Design review of the part built by this model. Coordinates are the model's own, in mm. A direction names the side the tool comes from. Give positions to 0.01 mm unless a question says otherwise; leave off trailing zeros. Order: outer loops, then holes, each group sorted by start corner. A loop starts at its lowest first (then second) coordinate and runs counter-clockwise, first axis right, second up.
```python
from build123d import *

# Parameters (mm, degrees)
SKETCH1_R           = 3.175
BOSS_EXTRUDE1_DEPTH = 20.6
SKETCH2_R           = 19.05
BOSS_EXTRUDE2_DEPTH = 1.6
BOSS_EXTRUDE3_DEPTH = 4.8
BOSS_EXTRUDE4_DEPTH = 51.2
SKETCH7_W           = 3.420526276
SKETCH7_H           = 1.112659396
CUT_EXTRUDE5_DEPTH  = 15
CUT_EXTRUDE6_REACH  = 70.749
SKETCH8_R           = 2.55
CUT_EXTRUDE7_DEPTH  = 17
CHAMFER1_SIZE       = 0.12
CHAMFER2_SIZE       = 0.4
SKETCH10_R          = 5.5
CUT_EXTRUDE8_DEPTH  = 5
BOSS_EXTRUDE5_START = 2.5
SKETCH11_R          = 3.175
BOSS_EXTRUDE5_DEPTH = 2.5
CHAMFER3_SIZE       = 0.4
CHAMFER4_SIZE       = 0.4
CUT_EXTRUDE9_START  = -1.6
SKETCH12_R          = 4
SKETCH12_R_2        = 3.175
CUT_EXTRUDE9_DEPTH  = 1.6


with BuildPart() as part:
    # Sketch1 → Boss-Extrude1 (new body)
    with BuildSketch(Plane.XY):
        with Locations(Location((0, 0, 0), (0, 0, 180))):
            Circle(SKETCH1_R)
    extrude(amount=BOSS_EXTRUDE1_DEPTH)

    # Sketch2 → Boss-Extrude2 (add)
    with BuildSketch(Plane(origin=(0, 0, 0), x_dir=(-1, 0, 0), z_dir=(0, 0, -1))):
        Circle(SKETCH2_R)
    extrude(amount=-BOSS_EXTRUDE2_DEPTH)

    # Sketch3 → Boss-Extrude3 (add)
    with BuildSketch(Plane(origin=(0, 0, 0), x_dir=(-1, 0, 0), z_dir=(0, 0, -1))):
        with BuildLine():
            Line((23.6, -28.2), (-23.6, -28.2))
            ThreePointArc((-23.6, -28.2), (-26.852691193, -26.852691193), (-28.2, -23.6))
            Line((-28.2, -23.6), (-28.2, 23.6))
            ThreePointArc((-28.2, 23.6), (-26.852691193, 26.852691193), (-23.6, 28.2))
            Line((-23.6, 28.2), (23.6, 28.2))
            ThreePointArc((23.6, 28.2), (26.852691193, 26.852691193), (28.2, 23.6))
            Line((28.2, 23.6), (28.2, -23.6))
            ThreePointArc((28.2, -23.6), (26.852691193, -26.852691193), (23.6, -28.2))
        make_face()
    extrude(amount=BOSS_EXTRUDE3_DEPTH)

    # Sketch4 → Boss-Extrude4 (add)
    with BuildSketch(Plane(origin=(0, 0, -4.8), x_dir=(-1, 0, 0), z_dir=(0, 0, -1))):
        with BuildLine():
            Line((-18.57, 23.57), (-18.57, 25.7))
            ThreePointArc((-18.57, 25.7), (-17.837766953, 27.467766953), (-16.07, 28.2))
            Line((-16.07, 28.2), (16.07, 28.2))
            ThreePointArc((16.07, 28.2), (17.837766953, 27.467766953), (18.57, 25.7))
            Line((18.57, 25.7), (18.57, 23.57))
            ThreePointArc((18.57, 23.57), (20.034466094, 20.034466094), (23.57, 18.57))
            Line((23.57, 18.57), (25.7, 18.57))
            ThreePointArc((25.7, 18.57), (27.467766953, 17.837766953), (28.2, 16.07))
            Line((28.2, 16.07), (28.2, -16.07))
            ThreePointArc((28.2, -16.07), (27.467766953, -17.837766953), (25.7, -18.57))
            Line((25.7, -18.57), (23.57, -18.57))
            ThreePointArc((23.57, -18.57), (20.034466094, -20.034466094), (18.57, -23.57))
            Line((18.57, -23.57), (18.57, -25.7))
            ThreePointArc((18.57, -25.7), (17.837766953, -27.467766953), (16.07, -28.2))
            Line((16.07, -28.2), (-16.07, -28.2))
            ThreePointArc((-16.07, -28.2), (-17.837766953, -27.467766953), (-18.57, -25.7))
            Line((-18.57, -25.7), (-18.57, -23.57))
            ThreePointArc((-18.57, -23.57), (-20.034466094, -20.034466094), (-23.57, -18.57))
            Line((-23.57, -18.57), (-25.7, -18.57))
            ThreePointArc((-25.7, -18.57), (-27.467766953, -17.837766953), (-28.2, -16.07))
            Line((-28.2, -16.07), (-28.2, 16.07))
            ThreePointArc((-28.2, 16.07), (-27.467766953, 17.837766953), (-25.7, 18.57))
            Line((-25.7, 18.57), (-23.57, 18.57))
            ThreePointArc((-23.57, 18.57), (-20.034466094, 20.034466094), (-18.57, 23.57))
        make_face()
    extrude(amount=BOSS_EXTRUDE4_DEPTH)

    # Sketch7 → Cut-Extrude5 (cut)
    with BuildSketch(Plane.XY.offset(20.6)):
        with Locations((0, 3.231329698)):
            Rectangle(SKETCH7_W, SKETCH7_H)
    extrude(amount=-CUT_EXTRUDE5_DEPTH, mode=Mode.SUBTRACT)

    # Sketch8 → Cut-Extrude6 (cut, up to next)
    with BuildSketch(Plane.XY, mode=Mode.PRIVATE) as cut_extrude6_sk1:
        with Locations((-23.57, 23.57)):
            Circle(SKETCH8_R)
    cut_extrude6_tool1 = extrude(cut_extrude6_sk1.sketch, amount=-CUT_EXTRUDE6_REACH, mode=Mode.PRIVATE) & part.part
    # Sketch8 → Cut-Extrude6 (cut, up to next)
    with BuildSketch(Plane.XY, mode=Mode.PRIVATE) as cut_extrude6_sk2:
        with Locations((23.57, 23.57)):
            Circle(SKETCH8_R)
    cut_extrude6_tool2 = extrude(cut_extrude6_sk2.sketch, amount=-CUT_EXTRUDE6_REACH, mode=Mode.PRIVATE) & part.part
    # Sketch8 → Cut-Extrude6 (cut, up to next)
    with BuildSketch(Plane.XY, mode=Mode.PRIVATE) as cut_extrude6_sk3:
        with Locations((23.57, -23.57)):
            Circle(SKETCH8_R)
    cut_extrude6_tool3 = extrude(cut_extrude6_sk3.sketch, amount=-CUT_EXTRUDE6_REACH, mode=Mode.PRIVATE) & part.part
    # Sketch8 → Cut-Extrude6 (cut, up to next)
    with BuildSketch(Plane.XY, mode=Mode.PRIVATE) as cut_extrude6_sk4:
        with Locations((-23.57, -23.57)):
            Circle(SKETCH8_R)
    cut_extrude6_tool4 = extrude(cut_extrude6_sk4.sketch, amount=-CUT_EXTRUDE6_REACH, mode=Mode.PRIVATE) & part.part
    add(cut_extrude6_tool1.solids().sort_by_distance((-23.57, 23.57, 0))[0], mode=Mode.SUBTRACT)
    add(cut_extrude6_tool2.solids().sort_by_distance((23.57, 23.57, 0))[0], mode=Mode.SUBTRACT)
    add(cut_extrude6_tool3.solids().sort_by_distance((23.57, -23.57, 0))[0], mode=Mode.SUBTRACT)
    add(cut_extrude6_tool4.solids().sort_by_distance((-23.57, -23.57, 0))[0], mode=Mode.SUBTRACT)

    # Sketch9 → Cut-Extrude7 (cut, symmetric)
    with BuildSketch(Plane.XY.offset(-28)):
        with BuildLine():
            Line((18.57, 23.57), (18.57, 25.7))
            ThreePointArc((18.57, 25.7), (17.837766953, 27.467766953), (16.07, 28.2))
            Line((16.07, 28.2), (-16.07, 28.2))
            ThreePointArc((-16.07, 28.2), (-17.837766953, 27.467766953), (-18.57, 25.7))
            Line((-18.57, 25.7), (-18.57, 23.57))
            ThreePointArc((-18.57, 23.57), (-20.034466094, 20.034466094), (-23.57, 18.57))
            Line((-23.57, 18.57), (-25.7, 18.57))
            ThreePointArc((-25.7, 18.57), (-27.467766953, 17.837766953), (-28.2, 16.07))
            Line((-28.2, 16.07), (-28.2, -16.07))
            ThreePointArc((-28.2, -16.07), (-27.467766953, -17.837766953), (-25.7, -18.57))
            Line((-25.7, -18.57), (-23.57, -18.57))
            ThreePointArc((-23.57, -18.57), (-20.034466094, -20.034466094), (-18.57, -23.57))
            Line((-18.57, -23.57), (-18.57, -25.7))
            ThreePointArc((-18.57, -25.7), (-17.837766953, -27.467766953), (-16.07, -28.2))
            Line((-16.07, -28.2), (16.07, -28.2))
            ThreePointArc((16.07, -28.2), (17.837766953, -27.467766953), (18.57, -25.7))
            Line((18.57, -25.7), (18.57, -23.57))
            ThreePointArc((18.57, -23.57), (20.034466094, -20.034466094), (23.57, -18.57))
            Line((23.57, -18.57), (25.7, -18.57))
            ThreePointArc((25.7, -18.57), (27.467766953, -17.837766953), (28.2, -16.07))
            Line((28.2, -16.07), (28.2, 16.07))
            ThreePointArc((28.2, 16.07), (27.467766953, 17.837766953), (25.7, 18.57))
            Line((25.7, 18.57), (23.57, 18.57))
            ThreePointArc((23.57, 18.57), (20.034466094, 20.034466094), (18.57, 23.57))
        make_face()
        with BuildLine():
            Line((18.47, 23.57), (18.47, 25.7))
            ThreePointArc((18.47, 25.7), (17.767056275, 27.397056275), (16.07, 28.1))
            Line((16.07, 28.1), (-16.07, 28.1))
            ThreePointArc((-16.07, 28.1), (-17.767056275, 27.397056275), (-18.47, 25.7))
            Line((-18.47, 25.7), (-18.47, 23.57))
            ThreePointArc((-18.47, 23.57), (-19.963755416, 19.963755416), (-23.57, 18.47))
            Line((-23.57, 18.47), (-25.7, 18.47))
            ThreePointArc((-25.7, 18.47), (-27.397056275, 17.767056275), (-28.1, 16.07))
            Line((-28.1, 16.07), (-28.1, -16.07))
            ThreePointArc((-28.1, -16.07), (-27.397056275, -17.767056275), (-25.7, -18.47))
            Line((-25.7, -18.47), (-23.57, -18.47))
            ThreePointArc((-23.57, -18.47), (-19.963755416, -19.963755416), (-18.47, -23.57))
            Line((-18.47, -23.57), (-18.47, -25.7))
            ThreePointArc((-18.47, -25.7), (-17.767056275, -27.397056275), (-16.07, -28.1))
            Line((-16.07, -28.1), (16.07, -28.1))
            ThreePointArc((16.07, -28.1), (17.767056275, -27.397056275), (18.47, -25.7))
            Line((18.47, -25.7), (18.47, -23.57))
            ThreePointArc((18.47, -23.57), (19.963755416, -19.963755416), (23.57, -18.47))
            Line((23.57, -18.47), (25.7, -18.47))
            ThreePointArc((25.7, -18.47), (27.397056275, -17.767056275), (28.1, -16.07))
            Line((28.1, -16.07), (28.1, 16.07))
            ThreePointArc((28.1, 16.07), (27.397056275, 17.767056275), (25.7, 18.47))
            Line((25.7, 18.47), (23.57, 18.47))
            ThreePointArc((23.57, 18.47), (19.963755416, 19.963755416), (18.47, 23.57))
        make_face(mode=Mode.SUBTRACT)
    extrude(amount=CUT_EXTRUDE7_DEPTH, both=True, mode=Mode.SUBTRACT)

    # Chamfer1
    chamfer1_edges = [part.edges().sort_by_distance(p)[0] for p in [
        (19.05, 0, 1.6),
    ]]
    chamfer(chamfer1_edges, length=CHAMFER1_SIZE)

    # Chamfer2
    chamfer2_edges = [part.edges().sort_by_distance(p)[0] for p in [
        (1.524883526, -2.784843843, 20.6),
    ]]
    chamfer(chamfer2_edges, length=CHAMFER2_SIZE)

    # Sketch10 → Cut-Extrude8 (cut)
    with BuildSketch(Plane(origin=(0, 0, -56), x_dir=(-1, 0, 0), z_dir=(0, 0, -1))):
        Circle(SKETCH10_R)
    extrude(amount=-CUT_EXTRUDE8_DEPTH, mode=Mode.SUBTRACT)

    # Sketch11 → Boss-Extrude5 (add)
    with BuildSketch(Plane(origin=(0, 0, -51), x_dir=(-1, 0, 0), z_dir=(0, 0, -1)).offset(BOSS_EXTRUDE5_START)):
        Circle(SKETCH11_R)
    extrude(amount=-BOSS_EXTRUDE5_DEPTH)

    # Chamfer3
    chamfer3_edges = [part.edges().sort_by_distance(p)[0] for p in [
        (3.175, 0, -53.5),
    ]]
    chamfer(chamfer3_edges, length=CHAMFER3_SIZE)

    # Chamfer4
    chamfer4_edges = [part.edges().sort_by_distance(p)[0] for p in [
        (5.5, 0, -56),
    ]]
    chamfer(chamfer4_edges, length=CHAMFER4_SIZE)

    # Sketch12 → Cut-Extrude9 (cut)
    with BuildSketch(Plane.XY.offset(1.6).offset(CUT_EXTRUDE9_START)):
        Circle(SKETCH12_R)
        with Locations(Location((0, 0, 0), (0, 0, 180))):
            Circle(SKETCH12_R_2, mode=Mode.SUBTRACT)
    extrude(amount=CUT_EXTRUDE9_DEPTH, mode=Mode.SUBTRACT)


solid = part.part
```
1. Draft analysis for pull direction X (two halves, no side actions). For faces 1 (the face through (-21.214, -24.547, -2.366)), 2 (the face through (17.786, 27.378, -27.762)), 3 (the face through (-0.12, -2.88, 20.49)), state which applies: pulls with the +X half, pulls with the -X half, needs draft (parallel to the pull), parting line crosses it, or undercut.
Recorded:
face 1: undercut
face 2: pulls with the +X half
face 3: parting line crosses it
2. For pin 1 (3 mm diameter, centred on x = -14, z = 4, fed in from +Y); pin 2 (0.6 mm diameter, centred on y = -25, z = -24.5, fed in from -X); pin 3 (1.1 mm diameter, centred on y = -25, z = -48, fed in from -X); pin 4 (0.6 mm diameter, centred on y = 24.5, z = -25, fed in from +X), all flat-tipped, find the tip position at first contact; note any pin that passes through.
Recorded:
pin 1: passes through
pin 2: stops at x = -18.47
pin 3: stops at x = -18.57
pin 4: stops at x = 18.47
3. Machinability: for faces 4 (the face through (-17.857, -27.448, -7.857)), 5 (the face through (17.857, 27.448, -7.857)), 6 (the face through (27.448, -17.857, -7.857)), 7 (the face through (-25, 18.57, -50)), 8 (the face through (-17.786, -27.378, -27.762)), which of the approach directions +Z, -Z, +X, -X, +Y, -Y give a long, thin tool a straight path to every point of the face, cutting with its end or side? Answer none if there is none.
Recorded:
face 4: -Z, -X, -Y
face 5: -Z, +X, +Y
face 6: -Z, +X, -Y
face 7: -Z, -X, +Y
face 8: -X, -Y
4. Take a section at C-C (z = 12.5). State the section outline as (x, y) points (3 decimals), then the cut area to 3 significant figures.
Recorded:
outline: (-1.71, 2.675) arc R3.175 ccw (long way) to (1.71, 2.675) - close
area: 30.5 mm2
5. Take a section at A-A (z = -8.5). State the section outline as (x, y) points, then the cut area to 3 significant figures.
Recorded:
outline: (-28.2, -16.07) arc R2.5 ccw to (-25.7, -18.57) - (-23.57, -18.57) arc R5 cw to (-18.57, -23.57) - (-18.57, -25.7) arc R2.5 ccw to (-16.07, -28.2) - (16.07, -28.2) arc R2.5 ccw to (18.57, -25.7) - (18.57, -23.57) arc R5 cw to (23.57, -18.57) - (25.7, -18.57) arc R2.5 ccw to (28.2, -16.07) - (28.2, 16.07) arc R2.5 ccw to (25.7, 18.57) - (23.57, 18.57) arc R5 cw to (18.57, 23.57) - (18.57, 25.7) arc R2.5 ccw to (16.07, 28.2) - (-16.07, 28.2) arc R2.5 ccw to (-18.57, 25.7) - (-18.57, 23.57) arc R5 cw to (-23.57, 18.57) - (-25.7, 18.57) arc R2.5 ccw to (-28.2, 16.07) - close
area: 2,820 mm2
6. Take a section at B-B (z = -41.5). State the section outline as (x, y) points, then the cut area to 3 significant figures.
Recorded:
outline: (-28.1, -16.07) arc R2.4 ccw to (-25.7, -18.47) - (-23.57, -18.47) arc R5.1 cw to (-18.47, -23.57) - (-18.47, -25.7) arc R2.4 ccw to (-16.07, -28.1) - (16.07, -28.1) arc R2.4 ccw to (18.47, -25.7) - (18.47, -23.57) arc R5.1 cw to (23.57, -18.47) - (25.7, -18.47) arc R2.4 ccw to (28.1, -16.07) - (28.1, 16.07) arc R2.4 ccw to (25.7, 18.47) - (23.57, 18.47) arc R5.1 cw to (18.47, 23.57) - (18.47, 25.7) arc R2.4 ccw to (16.07, 28.1) - (-16.07, 28.1) arc R2.4 ccw to (-18.47, 25.7) - (-18.47, 23.57) arc R5.1 cw to (-23.57, 18.47) - (-25.7, 18.47) arc R2.4 ccw to (-28.1, 16.07) - close
area: 2,800 mm2
7. For line 1 along Y through (x, z) = (-23.57, -2.7); line 2 along Y through (x, z) = (0, 1) (3 decimals); line 3 along Y through (x, z) = (0, -54.1), list the stretches that pass through material, from the lowest coordinate up.
Recorded:
line 1: y = -28.2 to -26.12, -21.02 to 21.02, 26.12 to 28.2
line 2: y = -19.05 to -4, -3.175 to 3.175, 4 to 19.05
line 3: y = -28.2 to -5.5, 5.5 to 28.2
